```python
from build123d import *

# Parameters (mm, degrees)
F0_W     = 800
F0_H     = 800
F1_DEPTH = 1
F2_R     = 270
F3_DEPTH = 3
F5_DEPTH = 1


with BuildPart() as f1:
    # F0 (on Front) → F1 (new body)
    with BuildSketch(Plane.XZ):
        Rectangle(F0_W, F0_H)
    extrude(amount=F1_DEPTH)

    # F2 (on Front) → F3 (cut)
    with BuildSketch(Plane.XZ):
        with Locations((0, -100)):
            Circle(F2_R)
    extrude(amount=F3_DEPTH, mode=Mode.SUBTRACT)

    # F4 (on face) → F5 (cut, through all)
    with BuildSketch(Plane.XZ.offset(1)):
        Polygon((250.5, -263), (227, -263), (227, -321), (285, -321), (285, -263), (261.5, -263), (261.5, -248), (250.5, -248), align=None)
        Polygon((320.098432, -173.013655), (297.615381, -179.851959), (293.250506, -165.501075), (282.726524, -168.701983), (287.091399, -183.052867), (264.608347, -189.89117), (281.485863, -245.381255), (336.975947, -228.50374), align=None)
        Polygon((327.492726, -76.708065), (307.972505, -89.792825), (299.62053, -77.333109), (290.483405, -83.457891), (298.83538, -95.917606), (279.315158, -109.002367), (311.609459, -157.179935), (359.787028, -124.885634), align=None)
        Polygon((306.542915, 17.581635), (291.674975, -0.617111), (280.058755, 8.873064), (273.099293, 0.354502), (284.715514, -9.135673), (269.847574, -27.334419), (314.763629, -64.02976), (351.45897, -19.113706), align=None)
        Polygon((259.062181, 101.694786), (250.133325, 79.957133), (236.258228, 85.656403), (232.078763, 75.481331), (245.95386, 69.782062), (237.025005, 48.044409), (290.675381, 26.007233), (312.712557, 79.65761), align=None)
        Polygon((189.159923, 168.351493), (186.942933, 144.956302), (172.009833, 146.371402), (170.972093, 135.420461), (185.905193, 134.005361), (183.688204, 110.61017), (241.429526, 105.138451), (246.901245, 162.879773), align=None)
        Polygon((102.886099, 211.782698), (107.572853, 188.754794), (92.874192, 185.763249), (95.067991, 174.98423), (109.766653, 177.975776), (114.453407, 154.947872), (171.288233, 166.51518), (159.720925, 223.350006), align=None)
        Polygon((7.707606, 228.229482), (18.892471, 207.561904), (5.7004, 200.422628), (10.935869, 190.748442), (24.12794, 197.887718), (35.312805, 177.22014), (86.322147, 204.825338), (58.716949, 255.834681), align=None)
        Polygon((-88.137971, 216.268396), (-71.423032, 199.749897), (-81.966754, 189.080787), (-74.14274, 181.348723), (-63.599017, 192.017833), (-46.884078, 175.499334), (-6.115017, 216.753227), (-47.368909, 257.522288), align=None)
        Polygon((-176.355311, 176.934657), (-155.556956, 165.994894), (-162.539784, 152.719348), (-152.804383, 147.598607), (-145.821556, 160.874153), (-125.023201, 149.93439), (-98.022934, 201.266501), (-149.355045, 228.266768), align=None)
        Polygon((-249.30931, 113.632553), (-226.227612, 109.218349), (-229.045189, 94.48535), (-218.240989, 92.419127), (-215.423412, 107.152126), (-192.341714, 102.737922), (-181.447083, 159.705518), (-238.414679, 170.60015), align=None)
        Polygon((-300.685885, 31.840807), (-277.318537, 34.334206), (-275.727006, 19.418878), (-264.789098, 20.586001), (-266.380629, 35.50133), (-243.013281, 37.994729), (-249.167203, 95.667333), (-306.839807, 89.513411), align=None)
        Polygon((-326.038455, -61.361604), (-304.407874, -52.176402), (-298.544979, -65.983156), (-288.420026, -61.6837), (-294.28292, -47.876946), (-272.652339, -38.691744), (-295.322198, 14.694373), (-348.708315, -7.975487), align=None)
        Polygon((-323.172786, -157.908122), (-305.151071, -142.826086), (-295.52424, -154.329308), (-287.088544, -147.269631), (-296.715375, -135.766409), (-278.693661, -120.684373), (-315.91741, -76.205248), (-360.396534, -113.428997), align=None)
        Polygon((-292.336897, -249.442761), (-279.483808, -229.769223), (-266.92623, -237.973322), (-260.909891, -228.764432), (-273.467468, -220.560333), (-260.614379, -200.886794), (-309.170346, -169.164277), (-340.892863, -217.720244), align=None)
        Polygon((-236.199598, -328.043307), (-229.627554, -305.480988), (-215.226074, -309.67591), (-212.149798, -299.114825), (-226.551278, -294.919903), (-219.979234, -272.357584), (-275.664957, -256.13722), (-291.885321, -311.822943), align=None)
    extrude(amount=-F5_DEPTH, mode=Mode.SUBTRACT)


solid = f1.part
```
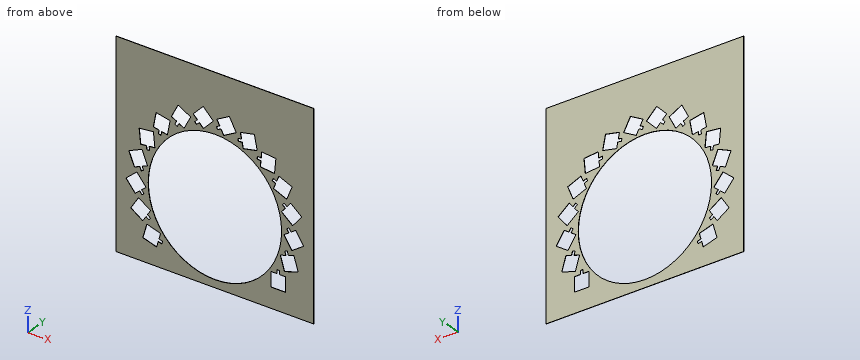
Can you work these out from the model? Positions are in its coordinate system, mm. Give positions to 0.01 mm unless a question says otherwise; leave off trailing zeros. Use a Markdown table: item, result. Add a question column.
Q1. I'm going to push a flat-ended pin straight in: pin 1 (5 mm diameter, centred on x = 261, z = -317, fed in from -Y). Where does the tip first touch, or does it pass through?
Q2. If we section it at A-A on y = -0.35: Count the separate pieces of the cut face and the enclosed holes in it, plus the area to 3 significant figures.
Q3. Please list where these lines run through material, in increasing order: line 1 along Z through (x, y) = (0, -0.4); line 2 along X through (y, z) = (-0.8, -2); line 3 along Z through (x, y) = (43, -0.75).
Answers follow:
| question | item | result |
|---|---|---|
| 1 | pin 1 | passes through |
| 2 | separate pieces | 1 |
| 2 | enclosed holes | 17 |
| 2 | area | 355,000 mm^2 |
| 3 | line 1 | z = -400 to -370, 170 to 400 |
| 3 | line 2 | x = -400 to -334.64, -288.23 to -251.59, 251.59 to 275.98, 330.51 to 400 |
| 3 | line 3 | z = -400 to -366.55, 166.55 to 181.38, 247.33 to 400 |
